The model under review builds one solid part; all positions refer to its coordinate system, in mm. A direction names the side the tool comes from. Round coordinates to 2 decimals unless told otherwise and drop trailing zeros. Order: outer loops, then holes, each group sorted by start corner. A loop starts at its lowest first (then second) coordinate and runs counter-clockwise, first axis right, second up.
1) Consider section A-A (x = -2.5). Give the boundary of the cut face in (y, z), then the cut area to 3 significant figures.
2) Consider section C-C (x = -35). Give the boundary of the cut face in (y, z), then the cut area to 3 significant figures.
3) Consider section B-B (z = 1.45). Give the boundary of the cut face in (x, y), then the cut area to 3 significant figures.
4) Mouldability with a two-part tool opening along X and no side actions: class faces 1 (the face through (-1, 4, 6)), 2 (the face through (36.99, 109.35, 3.04)) as pulls with the +X half, pulls with the -X half, needs draft (parallel to the pull), parting line crosses it, or undercut.
5) Machinability: for faces 3 (the face through (-36.99, 203.65, 3.04)), 4 (the face through (-1, 4, 0)), which of the approach directions +Z, -Z, +X, -X, +Y, -Y give a long, thin tool a straight path to every point of the face, cutting with its end or side? Answer none if there is none.
6) To check wall thickness, follow L1, parallel to Y at x = 16, z = 3.6; L2, parallel to X at y = 124, z = 0.9; L3, parallel to Y at x = -34, z = 4. State the ranges of each line that lie inside material, in increasing order.
Autodesk Inventor part; units mm, degrees
ref_plane "YZ Plane" through (0, 0, 0) normal (1, 0, 0) x (0, 1, 0)
ref_plane "XZ Plane" through (0, 0, 0) normal (0, 1, 0) x (-1, 0, 0)
ref_plane "XY Plane" through (0, 0, 0) normal (0, 0, 1) x (1, 0, 0)
sketch "Skizze1" plane through (0, 0, 0) normal (0, 0, 1) x (1, 0, 0)
  line L0 (0, 408.1) -> (0, -408.1)
  line L1 (-84.7, 0) -> (84.7, 0)
  line L2 (-60.5, -291.5) -> (60.5, -291.5)
  line L3 (60.5, -291.5) -> (60.5, 291.5)
  line L4 (60.5, 291.5) -> (-60.5, 291.5)
  line L5 (-60.5, 291.5) -> (-60.5, -291.5)
  point P0 (0, 0)
  point P1 (0, -291.5)
  point P2 (-60.5, 0)
  dimension "d0" = 583
  dimension "d1" = 121
extrude "Extrusion1" add sketch "Skizze1" along normal blind 6
sketch "Skizze2" plane through (0, 0, 0) normal (0, 0, -1) x (-1, 0, 0)
  line L0 (60.5, 291.5) -> (60.5, -291.5)
  line L1 (-60.5, 291.5) -> (60.5, 291.5)
  line L2 (-40, 106.5) -> (40, 106.5)
  line L3 (40, 106.5) -> (40, 206.5)
  line L4 (40, 206.5) -> (-40, 206.5)
  line L5 (-40, 206.5) -> (-40, 106.5)
  line L6 (50, 227.269) -> (50, 127.269)
  point P0 (0, 0)
  dimension "d4" = 185
  dimension "d5" = 100
  dimension "d6" = 80
  dimension "d7" = 20.5
extrude "Extrusion2" cut sketch "Skizze2" against normal through all
fillet "Rundung1" radius 10 4 edges at (-40, 106.5, 3) (-40, 206.5, 3) (40, 206.5, 3) (40, 106.5, 3)
properties part number "Schläuse" material "Polycarbonate, Clear"
Answer below:
1. outline: (-291.5, 0) - (106.5, 0) - (106.5, 6) - (-291.5, 6) - close; (206.5, 0) - (291.5, 0) - (291.5, 6) - (206.5, 6) - close
1. area: 2,900 mm2
2. outline: (-291.5, 0) - (107.84, 0) - (107.84, 6) - (-291.5, 6) - close; (205.16, 0) - (291.5, 0) - (291.5, 6) - (205.16, 6) - close
2. area: 2,910 mm2
3. outline: (-60.5, -291.5) - (60.5, -291.5) - (60.5, 291.5) - (-60.5, 291.5) - close; hole (-40, 116.5) arc R10 ccw to (-30, 106.5) - (30, 106.5) arc R10 ccw to (40, 116.5) - (40, 196.5) arc R10 ccw to (30, 206.5) - (-30, 206.5) arc R10 ccw to (-40, 196.5) - close
3. area: 62,600 mm2
4. face 1: needs draft
4. face 2: undercut
5. face 3: +Z, -Z
5. face 4: -Z, +X, -X, +Y, -Y
6. L1: y = -291.5 to 106.5, 206.5 to 291.5
6. L2: x = -60.5 to -40, 40 to 60.5
6. L3: y = -291.5 to 107.33, 205.67 to 291.5
